Geometry check sheet. Reference: the model listing, model coordinates, mm. A direction names the side the tool comes from. Coordinates: 2 decimals unless noted, no trailing zeros. Write each loop counter-clockwise with the first axis right and the second up, starting at its lowest first coordinate (ties: lowest second). Pieces come first, ordered by that corner, then holes. Notation, with made-up numbers: (-6, -33) -> (14, -33) arc R23 ccw to (14, -11) -> close; hole circle Ø5 at (-6, -35). An arc over 180 degrees is marked (long way). Put each result on its own line as item: value. Start each with the question number.
from build123d import *

# Parameters (mm, degrees)
SKETCH1_W               = 196.85
SKETCH1_H               = 50.8
BOSS_EXTRUDE1_DEPTH     = 6.35
SKETCH4_W               = 196.85
SKETCH4_H               = 6.35
CUT_EXTRUDE3_DEPTH      = 3.175
CUT_EXTRUDE1_DEPTH      = 1
CUT_EXTRUDE1_DEPTH_BACK = 51.8
CUT_EXTRUDE2_DEPTH      = 1
CUT_EXTRUDE2_DEPTH_BACK = 51.8


with BuildPart() as part:
    # Sketch1 → Boss-Extrude1 (new body)
    with BuildSketch(Plane(origin=(0, 0, 0), x_dir=(1, 0, 0), z_dir=(0, 1, 0))):
        Rectangle(SKETCH1_W, SKETCH1_H)
    extrude(amount=BOSS_EXTRUDE1_DEPTH)

    # Sketch4 → Cut-Extrude3 (cut)
    with BuildSketch(Plane(origin=(0, 6.35, 0), x_dir=(1, 0, 0), z_dir=(0, 1, 0))):
        with Locations((0, -15.875)):
            Rectangle(SKETCH4_W, SKETCH4_H)
    extrude(amount=-CUT_EXTRUDE3_DEPTH, mode=Mode.SUBTRACT)

    # Sketch2 → Cut-Extrude1 (cut, two sides)
    with BuildSketch(Plane.XY.offset(25.4)) as cut_extrude1_sk:
        Polygon((-384.028812745, -285.603812745), (-98.425, 0), (-92.075, 6.35), (193.528812745, 291.953812745), (-377.678812745, 863.161438235), (-955.236438235, 285.603812745), align=None)
    extrude(amount=CUT_EXTRUDE1_DEPTH, mode=Mode.SUBTRACT)
    extrude(cut_extrude1_sk.sketch, amount=-CUT_EXTRUDE1_DEPTH_BACK, mode=Mode.SUBTRACT)

    # Sketch3 → Cut-Extrude2 (cut, two sides)
    with BuildSketch(Plane.XY.offset(25.4)) as cut_extrude2_sk:
        Polygon((384.028812745, -285.603812745), (98.425, 0), (92.075, 6.35), (-193.528812745, 291.953812745), (377.678812745, 863.161438235), (955.236438235, 285.603812745), align=None)
    extrude(amount=CUT_EXTRUDE2_DEPTH, mode=Mode.SUBTRACT)
    extrude(cut_extrude2_sk.sketch, amount=-CUT_EXTRUDE2_DEPTH_BACK, mode=Mode.SUBTRACT)


solid = part.part
Item 1: Scan lines: line 1 along Z through (x, y) = (26.5, 4.75); line 2 along X through (y, z) = (3, -7.5) (3 decimals); line 3 along X through (y, z) = (4.5, 7.5) (3 decimals). Record each from-to range of solid material in increasing order. Write a range as [from, to].
Item 2: Access from +Z, -Z, +X, -X, +Y, -Y to the whole of each face (thin tool, end or side, straight path). Record for faces 4 (the flat face through (-1, 6.35, 22)), 5 (the flat face through (-1, 5, 19.05)).
Item 3: Mould release check, pull along Z, two halves, no side actions. Record for faces 1 (the flat face through (-1, 0, 0)), 2 (the flat face through (-1, 3, 25.4)), 3 (the flat face through (-1, 3.175, 16)): released by +Z, released by -Z, zero draft, split by the parting line, or undercut.
Item 4: Section check B-B, the plane x = -78. Enter the section's corners in (y, z) (3 decimals).
Item 5: Go/stop test with flat-tipped pins: P1, Ø1, axis at x = -60.5, z = 18.5, coming from the +Y side (3 decimals); P2, Ø10, axis at x = -24, z = -7.5, coming from the -Y side; P3, Ø1, axis at y = 2, z = 5.5, coming from the -X side (3 decimals). Record where each tip stops, or that it passes through.
Item 6: Section check D-D, the plane z = -13. Enter the section's corners in (x, y) (3 decimals).
Item 7: Section check A-A, the plane y = 5. Enter the section's corners in (x, z) (3 decimals), and give its area (3 significant figures).
Item 8: Section check C-C, the plane z = 15.5. Enter the section's corners in (x, y) (3 decimals), and give its area (3 significant figures).
From the geometry:
1. line 1: [-25.4, 12.7], [19.05, 25.4]
1. line 2: [-95.425, 95.425]
1. line 3: [-93.925, 93.925]
2. face 4: +Z, -Z, +X, -X, +Y
2. face 5: +X, -X, +Y
3. face 1: zero draft
3. face 2: released by +Z
3. face 3: undercut
4. outline: (0, -25.4) -> (6.35, -25.4) -> (6.35, 12.7) -> (3.175, 12.7) -> (3.175, 19.05) -> (6.35, 19.05) -> (6.35, 25.4) -> (0, 25.4) -> close
5. P1: y = 3.175
5. P2: y = 0
5. P3: x = -96.925
6. outline: (-98.425, 0) -> (98.425, 0) -> (92.075, 6.35) -> (-92.075, 6.35) -> close
7. outline: (-93.425, -25.4) -> (93.425, -25.4) -> (93.425, 12.7) -> (-93.425, 12.7) -> close; (-93.425, 19.05) -> (93.425, 19.05) -> (93.425, 25.4) -> (-93.425, 25.4) -> close
7. area: 8,310 mm²
8. outline: (-98.425, 0) -> (98.425, 0) -> (95.25, 3.175) -> (-95.25, 3.175) -> close
8. area: 615 mm²
